from build123d import *

# Parameters (mm, degrees)
SKETCH1_W               = 16
SKETCH1_H               = 16
BOSS_EXTRUDE1_DEPTH     = 55
SKETCH2_W               = 3
SKETCH2_H               = 16
CUT_EXTRUDE1_DEPTH      = 45
SKETCH3_R               = 3
CUT_EXTRUDE2_DEPTH      = 45
CUT_EXTRUDE3_DEPTH      = 35
FILLET1_R               = 5
FILLET2_R               = 3
CUT_EXTRUDE4_DEPTH      = 40
CUT_EXTRUDE4_DEPTH_BACK = 40
SKETCH5_R               = 1.75
CUT_EXTRUDE5_START      = -4
CUT_EXTRUDE5_DEPTH      = 40
CUT_EXTRUDE6_START      = -5
SKETCH7_R               = 3.5
CUT_EXTRUDE6_DEPTH      = 40


# Some blends are built 0.0001 mm under size
with BuildPart() as part:
    # Sketch1 → Boss-Extrude1 (new body)
    with BuildSketch(Plane.XY):
        Rectangle(SKETCH1_W, SKETCH1_H)
    extrude(amount=BOSS_EXTRUDE1_DEPTH)

    # Sketch2 → Cut-Extrude1 (cut)
    with BuildSketch(Plane(origin=(0, 8, 0), x_dir=(1, 0, 0), z_dir=(0, 1, 0))):
        with Locations((3, -8)):
            Rectangle(SKETCH2_W, SKETCH2_H)
        with Locations((-3, -8)):
            Rectangle(SKETCH2_W, SKETCH2_H)
    extrude(amount=-CUT_EXTRUDE1_DEPTH, mode=Mode.SUBTRACT)

    # Sketch3 → Cut-Extrude2 (cut)
    with BuildSketch(Plane(origin=(8, 0, 0), x_dir=(0, 0, -1), z_dir=(1, 0, 0))):
        with Locations((-6, 0)):
            Circle(SKETCH3_R)
    extrude(amount=-CUT_EXTRUDE2_DEPTH, mode=Mode.SUBTRACT)

    # Sketch4 → Cut-Extrude3 (cut)
    with BuildSketch(Plane.XY.offset(55)):
        with BuildLine():
            Line((0.5, 1.968626967), (0.5, 0.424558432))
            Line((0.5, 0.424558432), (-0.5, 0.424558432))
            Line((-0.5, 0.424558432), (-0.5, 1.968626967))
            ThreePointArc((-0.5, 1.968626967), (-2.645751311, -5), (4, -2))
            ThreePointArc((4, -2), (3, 0.645751311), (0.5, 1.968626967))
        make_face()
        with BuildLine():
            Line((-0.5, 0.424558432), (0.5, 0.424558432))
            Line((0.5, 0.424558432), (0.5, 1.968626967))
            ThreePointArc((0.5, 1.968626967), (0, 2), (-0.5, 1.968626967))
            Line((-0.5, 1.968626967), (-0.5, 0.424558432))
        make_face()
        with BuildLine():
            ThreePointArc((-0.5, 1.968626967), (0, 2), (0.5, 1.968626967))
            Line((0.5, 1.968626967), (0.5, 8))
            Line((0.5, 8), (-0.5, 8))
            Line((-0.5, 8), (-0.5, 1.968626967))
        make_face()
    extrude(amount=-CUT_EXTRUDE3_DEPTH, mode=Mode.SUBTRACT)

    # Fillet1
    fillet1_edges = [part.edges().sort_by_distance(p)[0] for p in [
        (8, 8, 27.5),
        (-8, 8, 27.5),
        (8, -8, 27.5),
        (-8, -8, 27.5),
    ]]
    fillet(fillet1_edges, radius=FILLET1_R - 0.0001)  # a hair under: the kernel refuses the full size

    # Fillet2
    # the kernel refuses this fillet: 3 mm, written as the material it takes off along each edge
    with BuildSketch(Plane(origin=(9, 8, 0), x_dir=(0, -1, 0), z_dir=(-1, 0, 0))) as fillet2_piece_1:
        with BuildLine():
            CenterArc((FILLET2_R, FILLET2_R), FILLET2_R, 180, 90)
            Line((0, FILLET2_R), (0, 0))
            Line((0, 0), (FILLET2_R, 0))
        make_face()
    extrude(amount=18, mode=Mode.SUBTRACT)
    with BuildSketch(Plane(origin=(-9, -8, 0), x_dir=(0, 0, 1), z_dir=(1, 0, 0))) as fillet2_piece_2:
        with BuildLine():
            CenterArc((FILLET2_R, -FILLET2_R), FILLET2_R, 90, 90)
            Line((0, -FILLET2_R), (0, 0))
            Line((0, 0), (FILLET2_R, 0))
        make_face()
    extrude(amount=18, mode=Mode.SUBTRACT)
    with BuildSketch(Plane(origin=(7, 8, 55), x_dir=(0, -1, 0), z_dir=(-1, 0, 0)), Plane(origin=(3.0001, 8, 55), x_dir=(0, -1, 0), z_dir=(-1, 0, 0))) as fillet2_piece_3:
        with BuildLine():
            CenterArc((FILLET2_R, -FILLET2_R), FILLET2_R, 90, 90)
            Line((0, -FILLET2_R), (0, 0))
            Line((0, 0), (FILLET2_R, 0))
        make_face()
    extrude(amount=10.0001, mode=Mode.SUBTRACT)
    with BuildSketch(Plane(origin=(8, -3.0001, 0), x_dir=(0, 0, 1), z_dir=(0, 1, 0)), Plane(origin=(8, -3.0001, 55), x_dir=(-1, 0, 0), z_dir=(0, 1, 0)), Plane(origin=(-8, 3.0001, 55), x_dir=(1, 0, 0), z_dir=(0, -1, 0))) as fillet2_piece_4:
        with BuildLine():
            CenterArc((FILLET2_R, -FILLET2_R), FILLET2_R, 90, 90)
            Line((0, -FILLET2_R), (0, 0))
            Line((0, 0), (FILLET2_R, 0))
        make_face()
    extrude(amount=6.0002, mode=Mode.SUBTRACT)
    with BuildSketch(Plane(origin=(3.0001, -3.0001, 0), x_dir=(-0.9304882617806061, -0.36632170927820573, 0), z_dir=(-0.36632170927820573, 0.9304882617806061, 0))) as fillet2_piece_5_section:
        with BuildLine():
            CenterArc((4.9999 - FILLET2_R, FILLET2_R), FILLET2_R, 270, 90)
            Line((4.9999 - FILLET2_R, 0), (4.9999, 0))
            Line((4.9999, 0), (4.9999, FILLET2_R))
        make_face()
    fillet2_piece_5 = revolve(axis=Axis((3.0001, -3.0001, 0), (0, 0, 1)), revolution_arc=158.511054393, mode=Mode.PRIVATE)
    fillet2_piece_5 = split(fillet2_piece_5, bisect_by=Plane(origin=(4.5, -5.386535126, 0.726343335), z_dir=(1, 0, 0)), keep=Keep.TOP, mode=Mode.PRIVATE)
    add(fillet2_piece_5, mode=Mode.SUBTRACT)
    with BuildSketch(Plane(origin=(3.0001, 3.0001, 0), x_dir=(1, 0, 0), z_dir=(0, -1, 0))) as fillet2_piece_6_section:
        with BuildLine():
            CenterArc((4.9999 - FILLET2_R, FILLET2_R), FILLET2_R, 270, 90)
            Line((4.9999 - FILLET2_R, 0), (4.9999, 0))
            Line((4.9999, 0), (4.9999, FILLET2_R))
        make_face()
    fillet2_piece_6 = revolve(axis=Axis((3.0001, 3.0001, 0), (0, 0, 1)), revolution_arc=158.511054393, mode=Mode.PRIVATE)
    fillet2_piece_6 = split(fillet2_piece_6, bisect_by=Plane(origin=(4.5, 5.386535107, 0.726343714), z_dir=(1, 0, 0)), keep=Keep.TOP, mode=Mode.PRIVATE)
    add(fillet2_piece_6, mode=Mode.SUBTRACT)
    with BuildSketch(Plane(origin=(-3.0001, -8, 55), x_dir=(0, 0, -1), z_dir=(1, 0, 0)), Plane(origin=(-8, 3.0001, 0), x_dir=(1, 0, 0), z_dir=(0, -1, 0))) as fillet2_piece_7:
        with BuildLine():
            CenterArc((FILLET2_R, FILLET2_R), FILLET2_R, 180, 90)
            Line((0, FILLET2_R), (0, 0))
            Line((0, 0), (FILLET2_R, 0))
        make_face()
    extrude(amount=6.0002, mode=Mode.SUBTRACT)
    with BuildSketch(Plane(origin=(-3.0001, -3.0001, 55), x_dir=(0, -1, 0), z_dir=(1, 0, 0))) as fillet2_piece_8:
        with BuildLine():
            CenterArc((4.9999 - FILLET2_R, FILLET2_R), FILLET2_R, 270, 90)
            Line((4.9999 - FILLET2_R, 0), (4.9999, 0))
            Line((4.9999, 0), (4.9999, FILLET2_R))
        make_face()
    revolve(axis=Axis((-3.0001, -3.0001, 55), (0, 0, -1)), revolution_arc=90, mode=Mode.SUBTRACT)
    with BuildSketch(Plane(origin=(3.0001, -3.0001, 55), x_dir=(0, -1, 0), z_dir=(-1, 0, 0))) as fillet2_piece_9:
        with BuildLine():
            CenterArc((4.9999 - FILLET2_R, -FILLET2_R), FILLET2_R, 0, 90)
            Line((4.9999, -FILLET2_R), (4.9999, 0))
            Line((4.9999, 0), (4.9999 - FILLET2_R, 0))
        make_face()
    revolve(axis=Axis((3.0001, -3.0001, 55), (0, 0, 1)), revolution_arc=90, mode=Mode.SUBTRACT)
    with BuildSketch(Plane(origin=(-3.0001, 3.0001, 55), x_dir=(-1, 0, 0), z_dir=(0, -1, 0))) as fillet2_piece_10:
        with BuildLine():
            CenterArc((4.9999 - FILLET2_R, FILLET2_R), FILLET2_R, 270, 90)
            Line((4.9999, FILLET2_R), (4.9999, 0))
            Line((4.9999, 0), (4.9999 - FILLET2_R, 0))
        make_face()
    revolve(axis=Axis((-3.0001, 3.0001, 55), (0, 0, -1)), revolution_arc=90, mode=Mode.SUBTRACT)
    with BuildSketch(Plane(origin=(3.0001, 3.0001, 55), x_dir=(1, 0, 0), z_dir=(0, -1, 0))) as fillet2_piece_11:
        with BuildLine():
            CenterArc((4.9999 - FILLET2_R, -FILLET2_R), FILLET2_R, 0, 90)
            Line((4.9999, -FILLET2_R), (4.9999, 0))
            Line((4.9999, 0), (4.9999 - FILLET2_R, 0))
        make_face()
    revolve(axis=Axis((3.0001, 3.0001, 55), (0, 0, 1)), revolution_arc=90, mode=Mode.SUBTRACT)
    with BuildSketch(Plane(origin=(-3.0001, -3.0001, 0), x_dir=(0.9304882617806057, -0.3663217092782066, 0), z_dir=(0.3663217092782066, 0.9304882617806057, 0))) as fillet2_piece_12_section:
        with BuildLine():
            CenterArc((4.9999 - FILLET2_R, -FILLET2_R), FILLET2_R, 0, 90)
            Line((4.9999 - FILLET2_R, 0), (4.9999, 0))
            Line((4.9999, 0), (4.9999, -FILLET2_R))
        make_face()
    fillet2_piece_12 = revolve(axis=Axis((-3.0001, -3.0001, 0), (0, 0, -1)), revolution_arc=158.511054393, mode=Mode.PRIVATE)
    fillet2_piece_12 = split(fillet2_piece_12, bisect_by=Plane(origin=(-4.5, -5.38653512, 0.72634326), z_dir=(-1, 0, 0)), keep=Keep.TOP, mode=Mode.PRIVATE)
    add(fillet2_piece_12, mode=Mode.SUBTRACT)
    with BuildSketch(Plane(origin=(-3.0001, 3.0001, 0), x_dir=(-1, 0, 0), z_dir=(0, -1, 0))) as fillet2_piece_13_section:
        with BuildLine():
            CenterArc((4.9999 - FILLET2_R, -FILLET2_R), FILLET2_R, 0, 90)
            Line((4.9999 - FILLET2_R, 0), (4.9999, 0))
            Line((4.9999, 0), (4.9999, -FILLET2_R))
        make_face()
    fillet2_piece_13 = revolve(axis=Axis((-3.0001, 3.0001, 0), (0, 0, -1)), revolution_arc=158.511054393, mode=Mode.PRIVATE)
    fillet2_piece_13 = split(fillet2_piece_13, bisect_by=Plane(origin=(-4.5, 5.386535101, 0.726343639), z_dir=(-1, 0, 0)), keep=Keep.TOP, mode=Mode.PRIVATE)
    add(fillet2_piece_13, mode=Mode.SUBTRACT)

    # Sketch5 → Cut-Extrude4 (cut, two sides: drawn at the far end of the back side and taken through both)
    with BuildSketch(Plane.ZY.offset(-0.5).offset(-CUT_EXTRUDE4_DEPTH_BACK)):
        with Locations(Location((48, 4.984313483, 0), (0, 0, 90))):
            Circle(SKETCH5_R)
        with Locations(Location((34, 4.984313483, 0), (0, 0, 90))):
            Circle(SKETCH5_R)
    extrude(amount=CUT_EXTRUDE4_DEPTH + CUT_EXTRUDE4_DEPTH_BACK, mode=Mode.SUBTRACT)

    # Sketch6 → Cut-Extrude5 (cut)
    with BuildSketch(Plane.ZY.offset(-0.5).offset(CUT_EXTRUDE5_START)):
        Polygon((49.674315781, 7.884313483), (46.325684219, 7.884313483), (44.651368439, 4.984313483), (46.325684219, 2.084313483), (49.674315781, 2.084313483), (51.348631561, 4.984313483), align=None)
        Polygon((35.885086056, 7.884313483), (32.536454495, 7.884313483), (30.862138714, 4.984313483), (32.536454495, 2.084313483), (35.885086056, 2.084313483), (37.559401836, 4.984313483), align=None)
    extrude(amount=-CUT_EXTRUDE5_DEPTH, mode=Mode.SUBTRACT)

    # Sketch7 → Cut-Extrude6 (cut)
    with BuildSketch(Plane(origin=(-0.5, 0, 0), x_dir=(0, 0, -1), z_dir=(1, 0, 0)).offset(CUT_EXTRUDE6_START)):
        with Locations((-48, 4.984313483)):
            Circle(SKETCH7_R)
        with Locations((-34, 4.984313483)):
            Circle(SKETCH7_R)
    extrude(amount=-CUT_EXTRUDE6_DEPTH, mode=Mode.SUBTRACT)


solid = part.part
Geometry: final body of the model. Coordinates: model frame, mm. A direction names the side the tool comes from. Coordinates: 2 decimals unless noted, no trailing zeros. Order: outer loops, then holes, each group sorted by start corner. A loop starts at its lowest first (then second) coordinate and runs counter-clockwise, first axis right, second up.
(1) Section query A-A (z = 34). Return the cut outline in (x, y).
(2) Section query D-D (x = 2). Return the cut outline in (y, z).
(3) First-contact query: pin 1 (5.5 mm diameter, centred on y = 4.98, z = 48, fed in from +X); pin 2 (1 mm diameter, centred on y = 5, z = 10.5, fed in from +X); pin 3 (2 mm diameter, centred on x = -4.5, z = 5.5, fed in from +Y). Flat tips, straight axial feed; report the tip coordinate or a pass-through.
(4) Access query for faces 5 (the face through (0.5, 5, 38)), 6 (the face through (-7.1, 0.04, 54.14)), 7 (the face through (5.68, 6.09, 31.5)), 8 (the face through (3, 0, 16)), 9 (the face through (-6.733, 1.486, 34.113)). Directions: +Z, -Z, +X, -X, +Y, -Y. A direction counts if a zero-diameter tool reaches every point of the face in a straight line with its end or side. Return the directions, or none.
(5) Material intervals for probe 1 along X at (y, z) = (3.75, 50.5); probe 2 along X at (y, z) = (-3, 13); probe 3 along Z at (x, y) = (5, 3.5), sorted ascending.
(6) Section query B-B (z = 6). State how many separate pieces and enclosed holes the cut face has, plus the area to 3 significant figures.
(7) Draft query along Z for faces 1 (the face through (-2.965, 4.605, 49.708)), 2 (the face through (4.5, 0, 10)), 3 (the face through (7.14, -0.04, 0.9)), 4 (the face through (6.23, 3.55, 31.69)). Return one class per face: pulls with the +Z half, pulls with the -Z half, needs draft (parallel to the pull), parting line crosses it, or undercut.
Solution:
1. outline: (-8, -3) arc R5 ccw to (-3, -8) - (3, -8) arc R5 ccw to (8, -3) - (8, 2.08) - (4.5, 2.08) - (4.5, 3.23) - (0.5, 3.23) - (0.5, 1.97) arc R4 cw (long way) to (-0.5, 1.97) - (-0.5, 3.23) - (-5.5, 3.23) - (-5.5, 1.48) - (-8, 1.48) - close; (-5.5, 6.73) - (-0.5, 6.73) - (-0.5, 8) - (-3, 8) arc R5 ccw to (-5.5, 7.33) - close; (0.5, 6.73) - (4.5, 6.73) - (4.5, 7.77) arc R5 ccw to (3, 8) - (0.5, 8) - close
2. outline: (-8, 16) - (8, 16) - (8, 52) arc R3 ccw to (5, 55) - (1.46, 55) - (1.46, 20) - (-5.46, 20) - (-5.46, 54.96) arc R3 ccw to (-8, 52) - close; hole circle Ø3.5 at (4.98, 34); hole circle Ø3.5 at (4.98, 48)
3. pin 1: stops at x = 4.5
3. pin 2: stops at x = 7.77
3. pin 3: stops at y = 7.77
4. face 5: +Z, +Y
4. face 6: +Z, -X, +Y, -Y
4. face 7: +X
4. face 8: -Z, +Y, -Y
4. face 9: -X
5. probe 1: x = -5.5 to -0.5, 0.5 to 4.5
5. probe 2: x = -8 to -4.5, -1.5 to 1.5, 4.5 to 8
5. probe 3: z = 0 to 31.72, 36.7 to 45.51, 50.49 to 55
6. separate pieces: 6
6. enclosed holes: 0
6. area: 79.0 mm2
7. face 1: undercut
7. face 2: needs draft
7. face 3: pulls with the -Z half
7. face 4: undercut
